For this review, take the finished solid that the model builds, in its own axes (mm). Coordinates: 2 decimals unless noted, no trailing zeros. Loops run counter-clockwise (first coordinate to the right, second up) from the corner with the lowest first, then second, coordinate; pieces in that order, holes last.
1. Take a section at B-B, the plane z = -0.75. State the section outline as (x, y) points, then the cut area to 3 significant figures.
2. Take a section at D-D, the plane z = 14.25. State the section outline as (x, y) points, then the cut area to 3 significant figures.
3. To check wall thickness, follow probe 1 along Z at (x, y) = (6, -0.5); probe 2 along Y at (x, z) = (0.5, 4); probe 3 along X at (y, z) = (-4.5, 11). State the ranges of each line that lie inside material, in increasing order.
4. Clearance check with flat-ended pins moving along their axes: P1, Ø1, axis at y = -4, z = 2, coming from the -X side; P2, Ø5, axis at y = 4.5, z = 12, coming from the -X side; P3, Ø5, axis at x = 6.5, z = 3, coming from the -Y side. State where each tip first meets the part, or that it passes through.
5. Take a section at A-A, the plane y = 0. State the section outline as (x, z) points.
6. Take a section at C-C, the plane x = 2.5. State the section outline as (y, z) points.
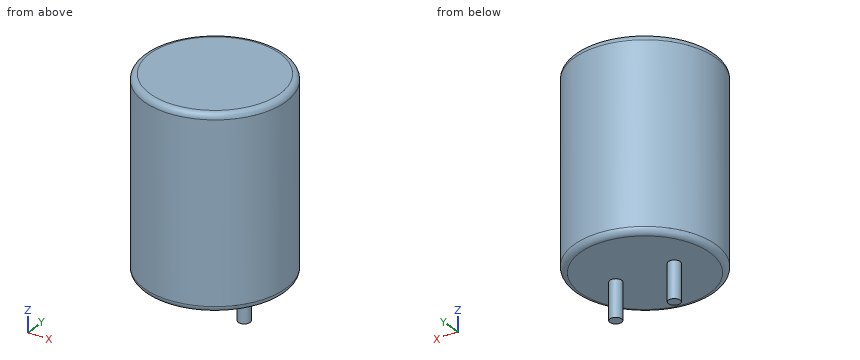
```python
from build123d import *

# Parameters (mm, degrees)
SKETCH001_R       = 0.5
PAD001_DEPTH      = 8
PAD001_DEPTH_BACK = 3.5
SKETCH_R          = 6
PAD_DEPTH         = 16
FILLET_R          = 0.5


with BuildPart() as pad001:
    # Sketch001 → Pad001 (new body, two sides)
    with BuildSketch(Plane.XY.offset(0.5)) as pad001_sk:
        Circle(SKETCH001_R)
        with Locations((5, 0)):
            Circle(SKETCH001_R)
    extrude(amount=PAD001_DEPTH)
    extrude(pad001_sk.sketch, amount=-PAD001_DEPTH_BACK)


with BuildPart() as obj1:
    # Sketch → Pad (new body)
    with BuildSketch(Plane.XY.offset(0.1)):
        with Locations((2.5, 0)):
            Circle(SKETCH_R)
    extrude(amount=PAD_DEPTH)

    # Fillet
    fillet_edges = [obj1.edges().sort_by_distance(p)[0] for p in [
        (-3.5, 0, 0.1),
        (-3.5, 0, 16.1),
    ]]
    fillet(fillet_edges, radius=FILLET_R)

    add(pad001.part)


solid = obj1.part
```
Results list:
1. outline: circle Ø1 at (0, 0); circle Ø1 at (5, 0)
1. area: 1.57 mm2
2. outline: circle Ø12 at (2.5, 0)
2. area: 113 mm2
3. probe 1: z = 0.1 to 16.1
3. probe 2: y = -5.66 to 5.66
3. probe 3: x = -1.47 to 6.47
4. P1: stops at x = -2.37
4. P2: stops at x = -3.16
4. P3: stops at y = -5.81
5. outline: (-3.5, 0.6) arc R0.5 ccw to (-3, 0.1) - (-0.5, 0.1) - (-0.5, -3) - (0.5, -3) - (0.5, 0.1) - (4.5, 0.1) - (4.5, -3) - (5.5, -3) - (5.5, 0.1) - (8, 0.1) arc R0.5 ccw to (8.5, 0.6) - (8.5, 15.6) arc R0.5 ccw to (8, 16.1) - (-3, 16.1) arc R0.5 ccw to (-3.5, 15.6) - close
6. outline: (-6, 0.6) arc R0.5 ccw to (-5.5, 0.1) - (5.5, 0.1) arc R0.5 ccw to (6, 0.6) - (6, 15.6) arc R0.5 ccw to (5.5, 16.1) - (-5.5, 16.1) arc R0.5 ccw to (-6, 15.6) - close
